Input: part model. Units: mm. Frame: model coordinates. Face numbers are marked on the shaded views. Round coordinates to 2 decimals unless told otherwise and drop trailing zeros. Loops run counter-clockwise (first coordinate to the right, second up) from the corner with the lowest first, then second, coordinate; pieces in that order, holes last. Notation, with made-up numbers: (2.5, 29) -> (21.5, 29) arc R16 cw to (21.5, 41) -> close; hole circle Ø8 at (78.25, 57.25). An arc over 180 degrees is marked (long way). Answer in a Markdown table with one row per item. Add a question column.
Q1. Ray query, L1, parallel to Y at x = 1.45, z = 0; L2, parallel to Y at x = 0.1, z = 0; L3, parallel to Z at x = 1.35, y = -2.25. Return the intervals inside material, ascending. Write a range as from..to.
Q2. Section A-A, the plane z = 0. Output: boundary loops of the cut face in (x, y).
Q3. Mould query, pull axis Z, two halves, no side actions, for the marked faces 1, 2 and 3. Classes: pulls with the +Z half, pulls with the -Z half, needs draft (parallel to the pull), parting line crosses it, or undercut.
Q4. Pin query (flat end, axial travel): pin 1 (1.5 mm diameter, centred on x = -1, z = -2, fed in from +Y); pin 2 (4.5 mm diameter, centred on y = 0, z = 0, fed in from +X). Return the tip coordinate at first contact, or that it passes through.
Q5. Section D-D, the plane y = -2.75. Output: boundary loops of the cut face in (x, z).
Q6. Section C-C, the plane x = -1.2. Output: boundary loops of the cut face in (y, z), and give its area (3 significant figures).
```python
from build123d import *

# Parameters (mm, degrees)
SKETCH1_R           = 4.5
SKETCH1_R_2         = 2.5
BOSS_EXTRUDE1_DEPTH = 1.5
SKETCH2_R           = 3.75
SKETCH2_R_2         = 3
CUT_EXTRUDE1_DEPTH  = 0.5


with BuildPart() as part:
    # Sketch1 → Boss-Extrude1 (new, symmetric)
    with BuildSketch(Plane(origin=(0, 0, 0), x_dir=(0, 0, -1), z_dir=(1, 0, 0))):
        Circle(SKETCH1_R)
        Circle(SKETCH1_R_2, mode=Mode.SUBTRACT)
    extrude(amount=BOSS_EXTRUDE1_DEPTH, both=True)

    # Sketch2 → Cut-Extrude1 (cut)
    with BuildSketch(Plane(origin=(1.5, 0, 0), x_dir=(0, 0, -1), z_dir=(1, 0, 0))):
        Circle(SKETCH2_R)
        Circle(SKETCH2_R_2, mode=Mode.SUBTRACT)
    extrude(amount=-CUT_EXTRUDE1_DEPTH, mode=Mode.SUBTRACT)


solid = part.part
```
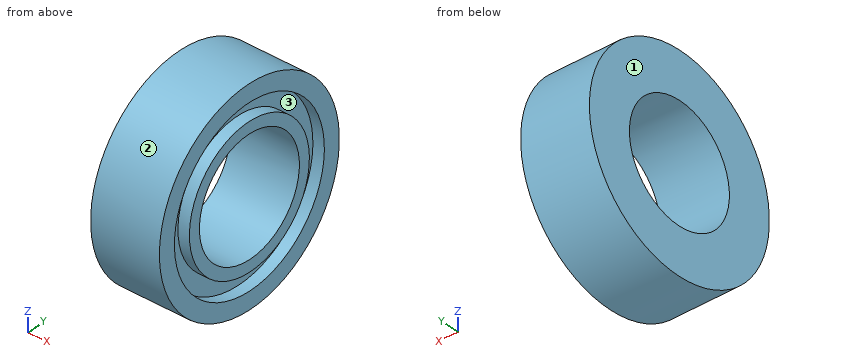
Answer block:
| question | item | result |
|---|---|---|
| 1 | L1 | -4.5..-3.75, -3..-2.5, 2.5..3, 3.75..4.5 |
| 1 | L2 | -4.5..-2.5, 2.5..4.5 |
| 1 | L3 | -3.9..-3, -1.98..-1.09, 1.09..1.98, 3..3.9 |
| 2 | outline | (-1.5, -4.5) -> (1.5, -4.5) -> (1.5, -3.75) -> (1, -3.75) -> (1, -3) -> (1.5, -3) -> (1.5, -2.5) -> (-1.5, -2.5) -> close; (-1.5, 2.5) -> (1.5, 2.5) -> (1.5, 3) -> (1, 3) -> (1, 3.75) -> (1.5, 3.75) -> (1.5, 4.5) -> (-1.5, 4.5) -> close |
| 3 | face 1 | needs draft |
| 3 | face 2 | parting line crosses it |
| 3 | face 3 | undercut |
| 4 | pin 1 | y = 4.32 |
| 4 | pin 2 | through |
| 5 | outline | (-1.5, -3.56) -> (1.5, -3.56) -> (1.5, -2.55) -> (1, -2.55) -> (1, -1.2) -> (1.5, -1.2) -> (1.5, 1.2) -> (1, 1.2) -> (1, 2.55) -> (1.5, 2.55) -> (1.5, 3.56) -> (-1.5, 3.56) -> close |
| 6 | outline | circle Ø9 at (0, 0); hole circle Ø5 at (0, 0) |
| 6 | area | 44.0 mm^2 |
